Build history of the part. All positions in model axes, mm. Coordinates: 2 decimals unless noted, no trailing zeros. Loops run counter-clockwise (first coordinate to the right, second up) from the corner with the lowest first, then second, coordinate; pieces in that order, holes last. Notation, with made-up numbers: (-35, -3) -> (-11, -3) arc R33 ccw to (-11, 28) -> close; hole circle Ø6 at (37.25, 49). An arc over 180 degrees is marked (long way). One line per item, written item: value. Start each with the question number.
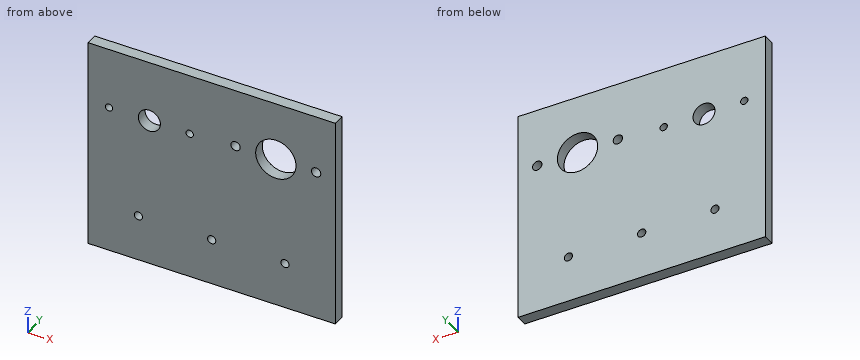
```python
from build123d import *

# Parameters (mm, degrees)
SKETCH1_W               = 65
SKETCH1_H               = 116
SKETCH1_W_2             = 70
BOSS_EXTRUDE1_DEPTH     = 6.35
F_10_CLEARANCE_HOLE1_D  = 5.1054
SKETCH9_R               = 11
CUT_EXTRUDE2_DEPTH      = 118.94309009
M4_CLEARANCE_HOLE1_D    = 4.5
CUT_EXTRUDE3_DEPTH      = 118.94309009
CUT_EXTRUDE3_DEPTH_BACK = 118.94309009
SKETCH12_R              = 6
SKETCH12_R_2            = 2


with BuildPart() as part:
    # Sketch1 → Boss-Extrude1 (new body)
    with BuildSketch(Plane(origin=(0, 0, 0), x_dir=(1, 0, 0), z_dir=(0, 1, 0))):
        Rectangle(SKETCH1_W, SKETCH1_H)
        with Locations((-67.5, 0)):
            Rectangle(SKETCH1_W_2, SKETCH1_H)
    extrude(amount=BOSS_EXTRUDE1_DEPTH)

    # #10 Clearance Hole1 (through all)
    with Locations(Plane(origin=(0, 6.35, 0), x_dir=(1, 0, 0), z_dir=(0, 1, 0))):
        with Locations((-22, -25.996), (22, -25.996)):
            Hole(F_10_CLEARANCE_HOLE1_D / 2)

    # Sketch9 → Cut-Extrude2 (cut, through all)
    with BuildSketch(Plane(origin=(0, 6.35, 0), x_dir=(1, 0, 0), z_dir=(0, 1, 0))):
        with Locations(Location((0, -25.996, 0), (0, 0, 270))):
            Circle(SKETCH9_R)
    extrude(amount=-CUT_EXTRUDE2_DEPTH, mode=Mode.SUBTRACT)

    # M4 Clearance Hole1 (through all)
    with Locations(Plane(origin=(0, 6.35, 0), x_dir=(1, 0, 0), z_dir=(0, 1, 0))):
        with Locations((-75, 32.6), (-35, 32.6), (5, 32.6)):
            Hole(M4_CLEARANCE_HOLE1_D / 2)

    # Sketch12 → Cut-Extrude3 (cut, two sides: drawn at the far end of the back side and taken through both)
    with BuildSketch(Plane(origin=(0, 6.35, 0), x_dir=(1, 0, 0), z_dir=(0, 1, 0)).offset(-CUT_EXTRUDE3_DEPTH_BACK)):
        with Locations(Location((-69, -24.5, 0), (0, 0, 270))):
            Circle(SKETCH12_R)
        with Locations(Location((-91, -24.5, 0), (0, 0, 270))):
            Circle(SKETCH12_R_2)
        with Locations(Location((-47, -24.5, 0), (0, 0, 270))):
            Circle(SKETCH12_R_2)
    extrude(amount=CUT_EXTRUDE3_DEPTH + CUT_EXTRUDE3_DEPTH_BACK, mode=Mode.SUBTRACT)


solid = part.part
```
Item 1: Band-saw the part on B-B, the plane x = 0. List the corners of the cut face in (y, z), and give its area (3 significant figures).
Item 2: Band-saw the part on D-D, the plane x = -35. List the corners of the cut face in (y, z).
Item 3: Band-saw the part on C-C, the plane y = 2. Count the separate pieces of the cut face and the enclosed holes in it, and give its area (3 significant figures).
Item 4: Probe probe 1 along X at (y, z) = (2.75, -32.6); probe 2 along Z at (x, y) = (22, 4.5); probe 3 along Z at (x, y) = (-35, 2.25). List the from-to ranges inside material, lowest first.
Item 5: Drop a flat-ended pin along its axis: pin 1 Ø6 at (x, z) = (-35, -32.6) entering from +Y. Give the stop position or say it passes through.
Item 6: Band-saw the part on A-A, the plane z = -32.6. List the corners of the cut face in (x, y).
Worked out:
1. outline: (0, -58) -> (6.35, -58) -> (6.35, 15) -> (0, 15) -> close; (0, 37) -> (6.35, 37) -> (6.35, 58) -> (0, 58) -> close
1. area: 597 mm²
2. outline: (0, -58) -> (6.35, -58) -> (6.35, -34.85) -> (0, -34.85) -> close; (0, -30.35) -> (6.35, -30.35) -> (6.35, 58) -> (0, 58) -> close
3. separate pieces: 1
3. enclosed holes: 9
3. area: 15,100 mm²
4. probe 1: x = -102.5 to -77.25, -72.75 to -37.25, -32.75 to 2.75, 7.25 to 32.5
4. probe 2: z = -58 to 23.44, 28.55 to 58
4. probe 3: z = -58 to -34.85, -30.35 to 58
5. pin 1: stops at y = 6.35
6. outline: (-102.5, 0) -> (-77.25, 0) -> (-77.25, 6.35) -> (-102.5, 6.35) -> close; (-72.75, 0) -> (-37.25, 0) -> (-37.25, 6.35) -> (-72.75, 6.35) -> close; (-32.75, 0) -> (2.75, 0) -> (2.75, 6.35) -> (-32.75, 6.35) -> close; (7.25, 0) -> (32.5, 0) -> (32.5, 6.35) -> (7.25, 6.35) -> close
